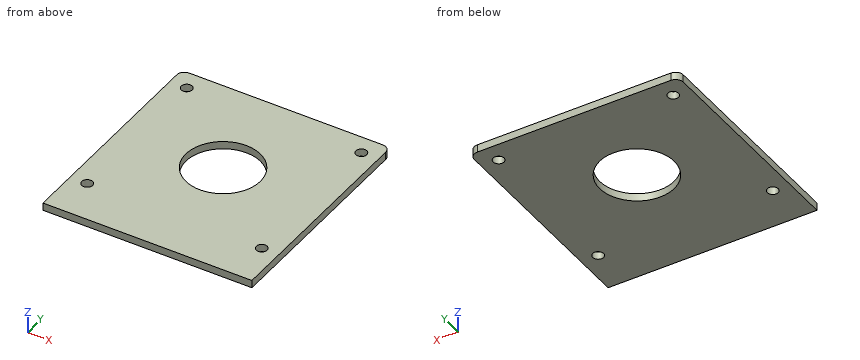
```python
from build123d import *

# Parameters (mm, degrees)
SKETCH2_W            = 86.36
SKETCH2_H            = 85.725
BOSS_EXTRUDE1_DEPTH  = 1.5875
SKETCH3_R            = 15.380999972
CUT_EXTRUDE1_DEPTH   = 61.924436241
M4_CLEARANCE_HOLE1_D = 4.5
SKETCH5_W            = 86.36
SKETCH5_H            = 6.35
BOSS_EXTRUDE2_DEPTH  = 3.175
FILLET1_R            = 3.175


with BuildPart() as part:
    # Sketch2 → Boss-Extrude1 (new, symmetric)
    with BuildSketch(Plane.XY):
        Rectangle(SKETCH2_W, SKETCH2_H)
    extrude(amount=BOSS_EXTRUDE1_DEPTH, both=True)

    # Sketch3 → Cut-Extrude1 (cut, through all)
    with BuildSketch(Plane.XY.offset(1.5875)):
        with Locations((-0.5, 1.8625)):
            Circle(SKETCH3_R)
    extrude(amount=-CUT_EXTRUDE1_DEPTH, mode=Mode.SUBTRACT)

    # M4 Clearance Hole1 (through all)
    with Locations(Plane(origin=(36.09137025, 34.95387025, 1.5875), x_dir=(1, 0, 0), z_dir=(0, 0, 1))):
        with Locations((0, 0), (0, -66.1827405), (-72.1827405, 0), (-72.1827405, -66.1827405)):
            Hole(M4_CLEARANCE_HOLE1_D / 2)

    # Sketch5 → Boss-Extrude2 (add)
    with BuildSketch(Plane.XY.offset(1.5875)):
        with Locations((0, -46.0375)):
            Rectangle(SKETCH5_W, SKETCH5_H)
    extrude(amount=-BOSS_EXTRUDE2_DEPTH)

    # Fillet1
    fillet1_edges = [part.edges().sort_by_distance(p)[0] for p in [
        (-43.18, 42.8625, 0),
        (43.18, 42.8625, 0),
    ]]
    fillet(fillet1_edges, radius=FILLET1_R)


solid = part.part
```
Geometry: final body of the model. Coordinates: model frame, mm. Round coordinates to 2 decimals unless told otherwise and drop trailing zeros. Write each loop counter-clockwise with the first axis right and the second up, starting at its lowest first coordinate (ties: lowest second). Pieces come first, ordered by that corner, then holes.
Item 1: Section query A-A (x = -35). Return loops of the section in (y, z), plus the area to 3 significant figures.
Item 2: Section query C-C (x = -0.5). Return loops of the section in (y, z).
Item 3: Section query D-D (y = 15). Return loops of the section in (x, z), plus the area to 3 significant figures.
Item 4: Material intervals for L1, parallel to X at y = -3, z = 1.1; L2, parallel to Y at x = -34.5, z = -1.05; L3, parallel to X at y = 12.5, z = 1.2, sorted ascending.
Item 5: Section query B-B (z = -0.85). Give the number of separate pieces and of enclosed holes in the cut face, plus the area to 3 significant figures.
Completed:
1. outline: (-49.21, -1.59) - (-33.2, -1.59) - (-33.2, 1.59) - (-49.21, 1.59) - close; (-29.26, -1.59) - (32.99, -1.59) - (32.99, 1.59) - (-29.26, 1.59) - close; (36.92, -1.59) - (42.86, -1.59) - (42.86, 1.59) - (36.92, 1.59) - close
1. area: 267 mm2
2. outline: (-49.21, -1.59) - (-13.52, -1.59) - (-13.52, 1.59) - (-49.21, 1.59) - close; (17.24, -1.59) - (42.86, -1.59) - (42.86, 1.59) - (17.24, 1.59) - close
3. outline: (-43.18, -1.59) - (-8.5, -1.59) - (-8.5, 1.59) - (-43.18, 1.59) - close; (7.5, -1.59) - (43.18, -1.59) - (43.18, 1.59) - (7.5, 1.59) - close
3. area: 223 mm2
4. L1: x = -43.18 to -15.09, 14.09 to 43.18
4. L2: y = -49.21 to -32.82, -29.64 to 33.36, 36.54 to 42.86
4. L3: x = -43.18 to -11.61, 10.61 to 43.18
5. separate pieces: 1
5. enclosed holes: 5
5. area: 7,140 mm2
